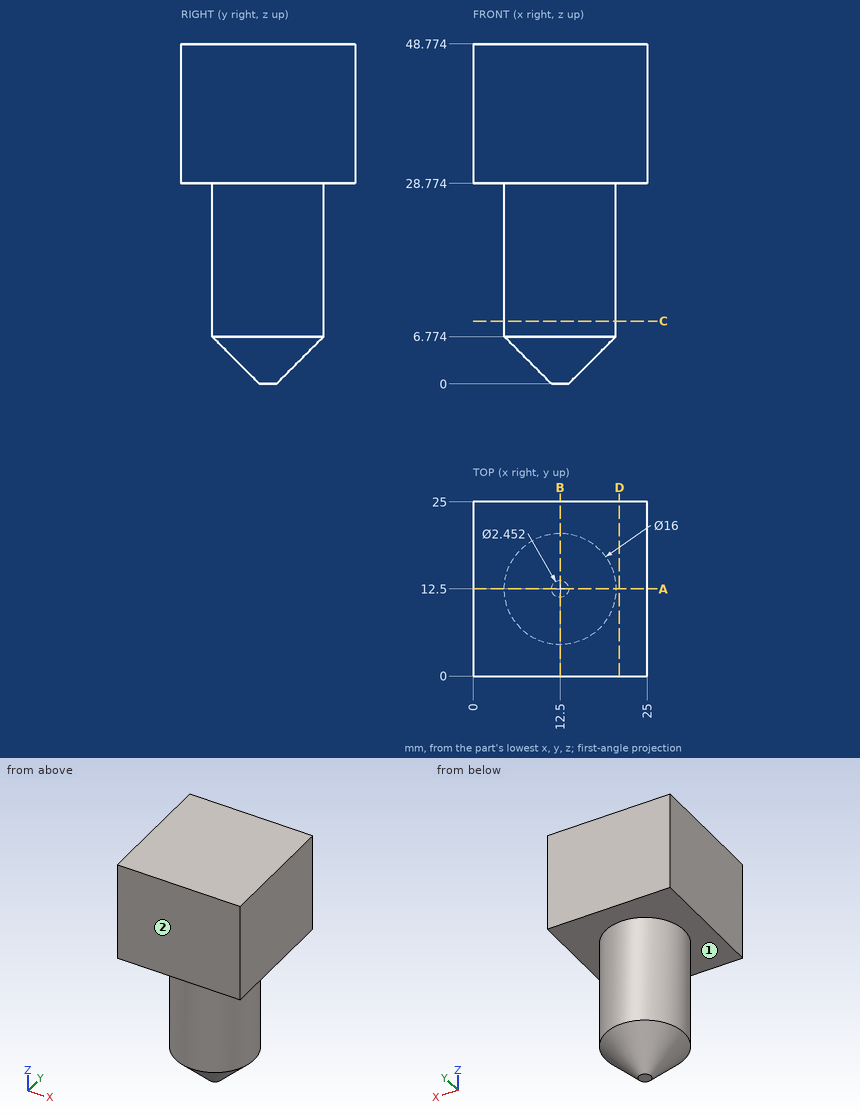
For this review, use the dimensioned drawing (mm, ordinates from the lowest corner) and the shaded views. A direction names the side the tool comes from. Round coordinates to 2 decimals unless told otherwise and drop trailing zeros. Write each loop counter-clockwise with the first axis right and the second up, starting at its lowest first coordinate (ties: lowest second). Pieces come first, ordered by that corner, then holes. Notation, with made-up numbers: M -9.5,83.5 L 31.5,83.5 A5 cw 31.5,88.5 Z; hole C 56.25,29 d4. An arc over 180 degrees is marked long. Use CSV: the item, a comma, the result in double quotes. Start each with the question number.
(1) We need section A-A, the plane y = 12.5. State the section outline as (x, z) points.
(2) Tool access review of the marked faces 1 and 2: name each direction out of +Z, -Z, +X, -X, +Y, -Y from which nothing blocks a thin tool from reaching the whole face with its end or side.
(3) We need section C-C, the plane z = 9. State the section outline as (x, y) points, then the cut area to 3 significant figures.
(4) For line 1 along Z through (x, y) = (23, 22); line 2 along Z through (x, y) = (10.75, 7.5) (1 decimal); line 3 along Y through (x, z) = (19.5, 27.5) (1 decimal), list the stretches that pass through material, from the lowest coordinate up.
(5) Clearance check with flat-ended pins moving along their axes: P1, Ø4, axis at x = 19.5, z = 20, coming from the +Y side (1 decimal); P2, Ø2, axis at x = 20.5, z = 17, coming from the -Y side (1 decimal); P3, Ø2, axis at x = 7.5, z = 31.5, coming from the -Y side; P4, Ø3, axis at x = 17, z = 10, coming from the -Y side. State where each tip first meets the part, or that it passes through.
(6) We need section D-D, the plane x = 21. State the section outline as (y, z) points, then the cut area to 3 significant figures.
Findings:
1,outline,"M 0,28.77 L 4.5,28.77 L 4.5,6.77 L 11.27,0 L 13.73,0 L 20.5,6.77 L 20.5,28.77 L 25,28.77 L 25,48.77 L 0,48.77 Z"
2,face 1,"-Z"
2,face 2,"+Z, -Z, +X, -X, -Y"
3,outline,"C 12.5,12.5 d16"
3,area,"201 mm^2"
4,line 1,"28.77 to 48.77"
4,line 2,"4.1 to 48.8"
4,line 3,"8.6 to 16.4"
5,P1,"y = 18.7"
5,P2,"y = 8.6"
5,P3,"y = 0"
5,P4,"y = 5.08"
6,outline,"M 0,28.77 L 25,28.77 L 25,48.77 L 0,48.77 Z"
6,area,"500 mm^2"
